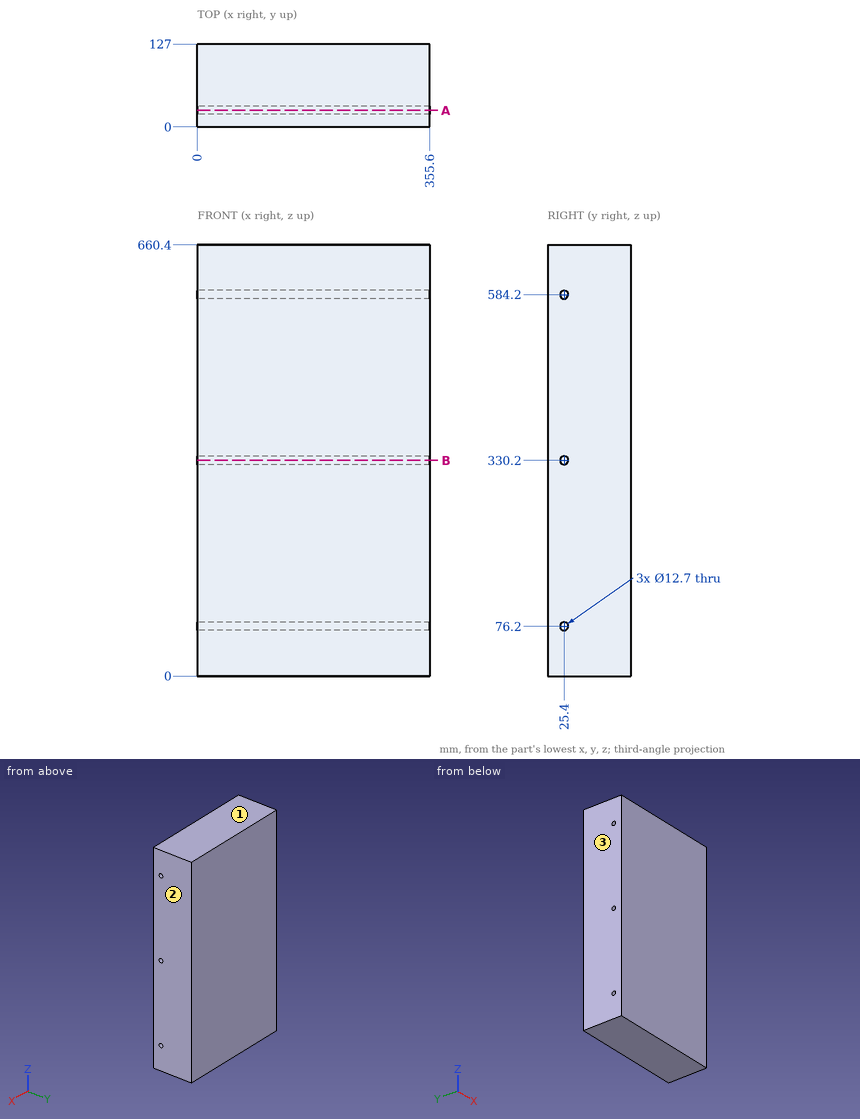
Study the drawing (mm; zero at the part's minimum x, y, z) and answer. Round coordinates to 2 decimals unless told otherwise and drop trailing zeros. Loops run counter-clockwise (first coordinate to the right, second up) from the corner with the lowest first, then second, coordinate; pieces in that order, holes last. Notation, with made-up numbers: (44, 74) - (74, 74) arc R32 ccw to (74, 101) - close; hole circle Ø8 at (-1, 61.25). An arc over 180 degrees is marked (long way). Use one line per item in the form item = value. Start each with the question number.
1. Given pin 1 Ø6 at (x, y) = (53, 65) entering from -Z; pin 2 Ø7.5 at (y, z) = (25.4, 584.2) entering from -X, each flat-ended and moving along its own axis, determine where each tip first touches the part or whether it passes through.
2. For a pull along X with two mould halves and no side action, classify the marked faces 1, 2 and 3 as pulls with the +X half, pulls with the -X half, needs draft (parallel to the pull), parting line crosses it, or undercut.
3. Consider line 1 (Z direction, x = 222, y = 25); line 2 (Y direction, x = 158, z = 330); line 3 (Y direction, x = 321, z = 74.5). Determine where each line is inside the solid, lowest interval first. Write a range as [from, to].
4. The part is cut by section B-B on z = 330.2. Determine the outline of the cut face in (x, y), then the cut area to 3 significant figures.
5. The part is cut by section A-A on y = 25.4. Determine the outline of the cut face in (x, z).
Geometry check:
q1.pin_1 = 0
q1.pin_2 = through
q2.face_1 = needs draft
q2.face_2 = pulls with the +X half
q2.face_3 = pulls with the -X half
q3.line_1 = [0, 69.86], [82.54, 323.86], [336.54, 577.86], [590.54, 660.4]
q3.line_2 = [0, 19.05], [31.75, 127]
q3.line_3 = [0, 19.28], [31.52, 127]
q4.outline = (0, 0) - (355.6, 0) - (355.6, 19.05) - (0, 19.05) - close; (0, 31.75) - (355.6, 31.75) - (355.6, 127) - (0, 127) - close
q4.area = 40,600 mm^2
q5.outline = (0, 0) - (355.6, 0) - (355.6, 69.85) - (0, 69.85) - close; (0, 82.55) - (355.6, 82.55) - (355.6, 323.85) - (0, 323.85) - close; (0, 336.55) - (355.6, 336.55) - (355.6, 577.85) - (0, 577.85) - close; (0, 590.55) - (355.6, 590.55) - (355.6, 660.4) - (0, 660.4) - close
